The listing builds one solid part. Answer for the finished solid, in the listing's coordinates (mm). A direction names the side the tool comes from. Round coordinates to 2 decimals unless told otherwise and drop trailing zeros. Order: outer loops, then holes, each group sorted by start corner. A loop starts at its lowest first (then second) coordinate and runs counter-clockwise, first axis right, second up. Notation, with made-up numbers: (70.25, -16) -> (104.25, -16) arc R17 ccw to (104.25, -11) -> close; hole circle Ø3 at (64.5, 65). An arc over 180 degrees is marked (long way). Return JSON: item names as keys, results as strings. Group by question number.
(1) Which of the six approach directions +Z, -Z, +X, -X, +Y, -Y give full straight-line access (tool end or side, diameter ignored) to faces 1 (the face through (-1.43, -17, 23.28)), 2 (the face through (-6, 15.5, 0)), 3 (the face through (-2, -20, -7.5))?
(2) The part is cut by section B-B (z = 0). Determine the outline of the cut face in (x, y), plus the area to 3 significant figures.
(3) The part is cut by section D-D (z = 22). Determine the outline of the cut face in (x, y).
(4) The part is cut by section C-C (x = 11). Determine the outline of the cut face in (y, z), plus the area to 3 significant figures.
(5) Consider line 1 (Y direction, x = 2.5, z = -6.5); line 2 (X direction, y = -9, z = 30.5); line 3 (Z direction, x = -2, y = 0). Determine where each line is inside the solid, lowest interval first. Write a range as [from, to].
(6) Determine the mould class of faces 4 (the face through (-7, -18.5, 23)), 5 (the face through (-2.166, -0.259, -31.302)), 6 (the face through (-1.521, 0.553, 4.214)) for opening direction Y: +Y half, -Y half, draft (parallel to the pull), parting line (faces both ways), or undercut.
(7) Each of these flat-tipped pins is pushed along its axis until it touches: pin 1 (2.5 mm diameter, centred on x = -6.5, z = -4, fed in from -Y); pin 2 (4 mm diameter, centred on x = -2.5, z = 21.5, fed in from +Y); pin 3 (0.9 mm diameter, centred on x = -1.5, y = -21, fed in from -Z). Where does it stop, or does it pass through?
(8) The part is cut by section A-A (y = 0). Determine the outline of the cut face in (x, z).
from build123d import *

# Parameters (mm, degrees)
EXTRUSION1_DEPTH         = 35
ENL_V_MAT_EXTRU_1_DEPTH  = 45.036916332
ESQUISSE8_W              = 15
ESQUISSE8_H              = 3
ENL_V_MAT_EXTRU_8_DEPTH  = 44.591857038
ESQUISSE9_W              = 23.50235156
ESQUISSE9_H              = 7
ENL_V_MAT_EXTRU_9_DEPTH  = 44.591857038
ESQUISSE11_R             = 2.1
EXTRUSION2_DEPTH         = 3
ESQUISSE12_R             = 4.25
ENL_V_MAT_EXTRU_10_DEPTH = 48.699580711
CONG_3_R                 = 2
CONG_4_R                 = 5
ENL_V_MAT_EXTRU_11_DEPTH = 47.521500481


with BuildPart() as part:
    # Esquisse1 → Extrusion1 (new, symmetric)
    with BuildSketch(Plane.XY):
        Polygon((-8, 18.5), (0, 18.5), (0, -25.5), (-3, -25.5), (-3, -18.5), (-8, -18.5), (-8, -15.5), (-3, -15.5), (-3, 15.5), (-8, 15.5), align=None)
    extrude(amount=EXTRUSION1_DEPTH, both=True)

    # Esquisse2 → Enlèv. mat.-Extru.1 (cut, through all)
    with BuildSketch(Plane.ZY.offset(8)):
        with BuildLine():
            Line((-11.49764844, -25.5), (-11.49764844, -14.49882422))
            ThreePointArc((-11.49764844, -14.49882422), (-9.49882422, -12.5), (-7.5, -14.49882422))
            Line((-7.5, -14.49882422), (-7.5, -25.5))
            Line((-7.5, -25.5), (-11.49764844, -25.5))
        make_face()
        with BuildLine():
            Line((7.5, -25.5), (7.5, -14.49882422))
            ThreePointArc((7.5, -14.49882422), (9.49882422, -12.5), (11.49764844, -14.49882422))
            Line((11.49764844, -14.49882422), (11.49764844, -25.5))
            Line((11.49764844, -25.5), (7.5, -25.5))
        make_face()
    extrude(amount=-ENL_V_MAT_EXTRU_1_DEPTH, mode=Mode.SUBTRACT)

    # Esquisse8 → Enlèv. mat.-Extru.8 (cut, through all)
    with BuildSketch(Plane.ZY.offset(3)):
        with Locations((0, -17)):
            Rectangle(ESQUISSE8_W, ESQUISSE8_H)
    extrude(amount=ENL_V_MAT_EXTRU_8_DEPTH, mode=Mode.SUBTRACT)

    # Esquisse9 → Enlèv. mat.-Extru.9 (cut, through all)
    with BuildSketch(Plane.ZY.offset(3)):
        with Locations((-23.24882422, -22)):
            Rectangle(ESQUISSE9_W, ESQUISSE9_H)
        with Locations((23.24882422, -22)):
            Rectangle(ESQUISSE9_W, ESQUISSE9_H)
    extrude(amount=-ENL_V_MAT_EXTRU_9_DEPTH, mode=Mode.SUBTRACT)

    # Esquisse11 → Extrusion2 (add)
    with BuildSketch(Plane.XZ.offset(25.5)):
        with BuildLine():
            Line((0, 7.5), (11.783181352, 5.948665982))
            ThreePointArc((11.783181352, 5.948665982), (17, 0), (11.783181352, -5.948665982))
            Line((11.783181352, -5.948665982), (0, -7.5))
            Line((0, -7.5), (0, 7.5))
        make_face()
        with Locations(Location((11, 0, 0), (0, 0, 270))):
            Circle(ESQUISSE11_R, mode=Mode.SUBTRACT)
    extrude(amount=-EXTRUSION2_DEPTH)

    # Esquisse12 → Enlèv. mat.-Extru.10 (cut, through all)
    with BuildSketch(Plane.ZY.offset(3)):
        with Locations(Location((0, 0, 0), (0, 0, 270))):
            Circle(ESQUISSE12_R)
    extrude(amount=-ENL_V_MAT_EXTRU_10_DEPTH, mode=Mode.SUBTRACT)

    # Congé3
    cong_3_edges = [part.edges().sort_by_distance(p)[0] for p in [
        (0, -22.5, 0),
        (-3, -15.5, 23.24882422),
        (-3, 15.5, 0),
        (-3, -15.5, -23.24882422),
    ]]
    fillet(cong_3_edges, radius=CONG_3_R)

    # Congé4
    cong_4_edges = [part.edges().sort_by_distance(p)[0] for p in [
        (0, -18.5, -23.24882422),
        (0, -18.5, 23.24882422),
        (0, 18.5, 0),
        (-3, -25.5, 0),
    ]]
    fillet(cong_4_edges, radius=CONG_4_R)

    # Esquisse13 → Enlèv. mat.-Extru.11 (cut, through all)
    with BuildSketch(Plane(origin=(0, 0, 0), x_dir=(0, 0, -1), z_dir=(1, 0, 0))):
        Polygon((-35, 18.5), (-35, -18.5), (-27.5, 18.5), align=None)
        Polygon((35, 18.5), (35, -18.5), (27.5, 18.5), align=None)
    extrude(amount=-ENL_V_MAT_EXTRU_11_DEPTH, mode=Mode.SUBTRACT)


solid = part.part
Answer below:
{
 "1": {"face 1": "+Z, +X, -Y", "face 2": "+Z, -Z, -X", "face 3": "+X, -X, -Y"},
 "2": {"outline": "(-8, 15.5) -> (-5, 15.5) arc R2 cw to (-3, 13.5) -> (-3, 4.25) -> (0, 4.25) -> (0, 13.5) arc R5 ccw to (-5, 18.5) -> (-8, 18.5) -> close; (-3, -20.5) arc R5 ccw to (2, -25.5) -> (8.9, -25.5) -> (8.9, -22.5) -> (2, -22.5) arc R2 cw to (0, -20.5) -> (0, -4.25) -> (-3, -4.25) -> close; (13.1, -25.5) -> (17, -25.5) -> (17, -22.5) -> (13.1, -22.5) -> close", "area": "151 mm²"},
 "3": {"outline": "(-8, -18.5) -> (-5, -18.5) arc R5 ccw to (0, -13.5) -> (0, 13.5) arc R5 ccw to (-5, 18.5) -> (-8, 18.5) -> (-8, 15.5) -> (-5, 15.5) arc R2 cw to (-3, 13.5) -> (-3, -13.5) arc R2 cw to (-5, -15.5) -> (-8, -15.5) -> close"},
 "4": {"outline": "(-25.5, -6.05) -> (-22.5, -6.05) -> (-22.5, -2.1) -> (-25.5, -2.1) -> close; (-25.5, 2.1) -> (-22.5, 2.1) -> (-22.5, 6.05) -> (-25.5, 6.05) -> close", "area": "23.7 mm²"},
 "5": {"line 1": "y = [-25.5, -22.5]", "line 2": "x = [-3, 0]", "line 3": "z = [-31.25, -4.25], [4.25, 31.25]"},
 "6": {"face 4": "-Y half", "face 5": "+Y half", "face 6": "undercut"},
 "7": {"pin 1": "stops at y = 15.5", "pin 2": "stops at y = 18.47", "pin 3": "stops at z = -7.5"},
 "8": {"outline": "(-3, -31.25) -> (0, -31.25) -> (0, -4.25) -> (-3, -4.25) -> close; (-3, 4.25) -> (0, 4.25) -> (0, 31.25) -> (-3, 31.25) -> close"}
}
